Design review of the part built by this model. Coordinates are the model's own, in mm. Round coordinates to 2 decimals unless told otherwise and drop trailing zeros. Loops run counter-clockwise (first coordinate to the right, second up) from the corner with the lowest first, then second, coordinate; pieces in that order, holes last. Notation, with made-up numbers: (48, 32.5) - (105, 32.5) arc R35 ccw to (105, 69.5) - close; hole circle Ø2 at (30, 1.5). An arc over 180 degrees is marked (long way). Answer as CSV lines item,"result". Start each with the question number.
(1) Mouldability with a two-part tool opening along X and no side actions: class faces 1 (the cylindrical face through (4.13, 7.21, 2.44)), 2 (the cylindrical face through (-4.13, 7.21, -2.44)), 3 (the cylindrical face through (-1.93, 3.91, -2.52)), 4 (the flat face through (0, 3, 5.556)) as released by +X, released by -X, zero draft, split by the parting line, or undercut.
(2) Consider section C-C (y = 7). Give the boundary of the cut face in (x, z) (3 decimals).
(3) Wall thickness on L1, parallel to Z at x = 0, y = 3.25 (3 decimals); L2, parallel to Z at x = -1, y = 3.5; L3, parallel to X at y = 1.5, z = 1: over which ranges is each line inside the solid? List them lowest first.
(4) For P1, Ø3, axis at y = 1.5, z = 4, coming from the -X side; P2, Ø2, axis at x = -1, z = 0, coming from the +Y side; P3, Ø3, axis at y = 6.5, z = -3.5, coming from the +X side, all flat-tipped, find the tip position at first contact; note any pin that passes through.
(5) Consider section B-B (x = 0.5). Give the boundary of the cut face in (y, z), and give its area (3 significant figures).
(6) Consider section A-A (y = 0.5). Give the boundary of the cut face in (x, z) (3 decimals), and give its area (3 significant figures).
from build123d import *

# Parameters (mm, degrees)
SKETCH1_R           = 3.175
BOSS_EXTRUDE1_DEPTH = 7.9375
FILLET1_R           = 2.54


with BuildPart() as part:
    # Sketch1 → Boss-Extrude1 (new body)
    with BuildSketch(Plane(origin=(0, 0, 0), x_dir=(1, 0, 0), z_dir=(0, 1, 0))):
        Polygon((-6.415804866, 0), (-3.207902433, -5.55625), (3.207902433, -5.55625), (6.415804866, 0), (3.207902433, 5.55625), (-3.207902433, 5.55625), align=None)
        with Locations(Location((0, 0, 0), (0, 0, 270))):
            Circle(SKETCH1_R, mode=Mode.SUBTRACT)
    extrude(amount=BOSS_EXTRUDE1_DEPTH)

    # Fillet1
    # the kernel refuses this fillet: 2.54 mm, written as the material it takes off along each edge
    with BuildSketch(Plane(origin=(-9.557902433, 7.9375, 5.55625), x_dir=(0, -1, 0), z_dir=(1, 0, 0)), Plane(origin=(0.032902433, 7.9375, 11.055511314), x_dir=(0, -1, 0), z_dir=(0.49999999999999967, 0, -0.8660254037844389)), Plane(origin=(9.590804866, 7.9375, 5.499261314), x_dir=(0, -1, 0), z_dir=(-0.5000000000000002, 0, -0.8660254037844386)), Plane(origin=(9.557902433, 7.9375, -5.55625), x_dir=(0, -1, 0), z_dir=(-1, 0, 0)), Plane(origin=(-0.032902433, 7.9375, -11.055511314), x_dir=(0, -1, 0), z_dir=(-0.49999999999999983, 0, 0.8660254037844388)), Plane(origin=(-9.590804866, 7.9375, -5.499261314), x_dir=(0, -1, 0), z_dir=(0.5000000000000001, 0, 0.8660254037844386))) as fillet1_piece_1:
        with BuildLine():
            CenterArc((FILLET1_R, FILLET1_R), FILLET1_R, 180, 90)
            Line((0, FILLET1_R), (0, 0))
            Line((0, 0), (FILLET1_R, 0))
        make_face()
    extrude(amount=19.115804866, mode=Mode.SUBTRACT)


solid = part.part
Determined:
1,face 1,"released by +X"
1,face 2,"released by -X"
1,face 3,"undercut"
1,face 4,"zero draft"
2,outline,"(-5.758, 0) - (-2.879, -4.987) - (2.879, -4.987) - (5.758, 0) - (2.879, 4.987) - (-2.879, 4.987) - close; hole circle Ø6.35 at (0, 0)"
3,L1,"z = -5.556 to -3.175, 3.175 to 5.556"
3,L2,"z = -5.56 to -3.01, 3.01 to 5.56"
3,L3,"x = -5.84 to -3.01, 3.01 to 5.84"
4,P1,"stops at x = -4.97"
4,P2,"passes through"
4,P3,"stops at x = 5.13"
5,outline,"(0, -5.56) - (5.4, -5.56) arc R2.54 ccw to (7.93, -3.14) - (0, -3.14) - close; (0, 3.14) - (7.93, 3.14) arc R2.54 ccw to (5.4, 5.56) - (0, 5.56) - close"
5,area,"35.7 mm^2"
6,outline,"(-6.416, 0) - (-3.208, -5.556) - (3.208, -5.556) - (6.416, 0) - (3.208, 5.556) - (-3.208, 5.556) - close; hole circle Ø6.35 at (0, 0)"
6,area,"75.3 mm^2"
